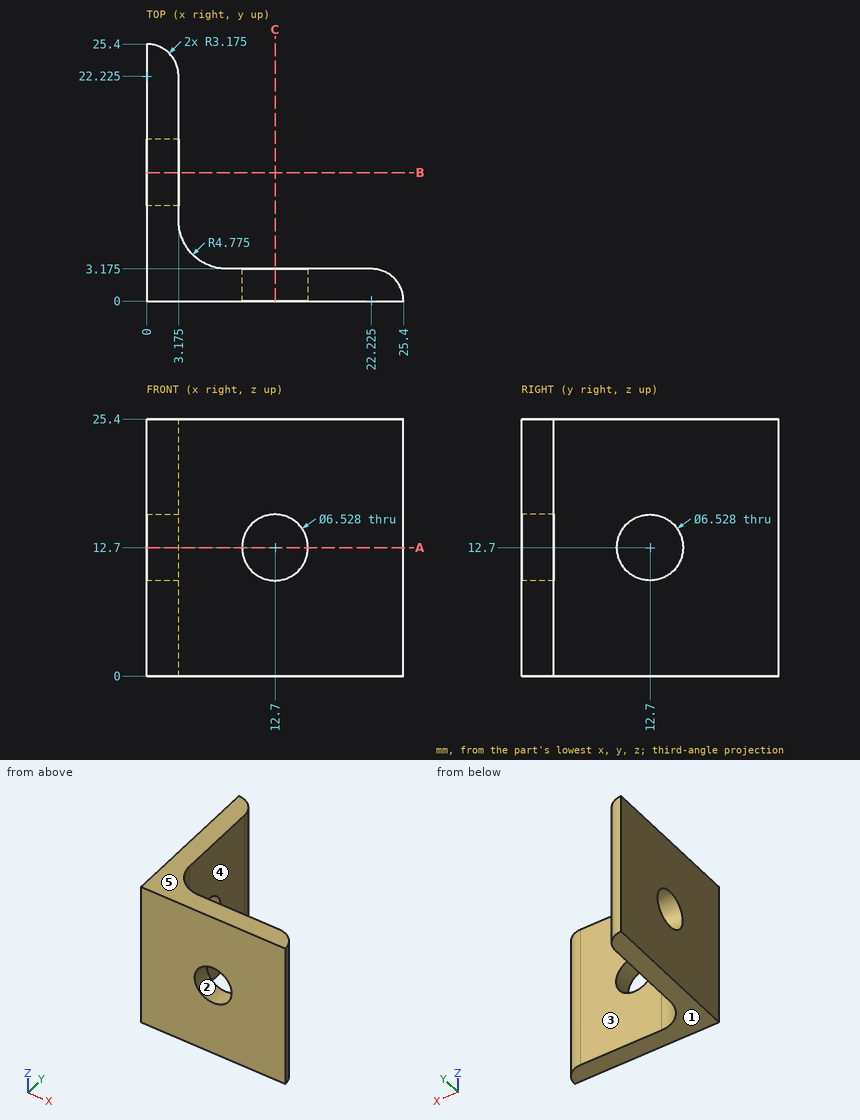
Could you check a few things on this drawing? It's one solid part, dimensions in mm from its lowest x, y, z. A direction names the side the tool comes from. Coordinates: 2 decimals unless noted, no trailing zeros. Loops run counter-clockwise (first coordinate to the right, second up) from the corner with the lowest first, then second, coordinate; pieces in that order, holes last.
1. For the marked faces 4 and 5, which set-ups out of +Z, -Z, +X, -X, +Y, -Y let a thin tool reach every point of the face, with its end or its side?
2. Imagine slicing it at B-B (y = 12.7). Please give me the cut outline in (x, z) (1 decimal).
3. I need wall thicknesses on L1, parallel to Z at x = 12.7, y = 2.15; L2, parallel to Y at x = 0.7, z = 12.7; L3, parallel to Y at x = 15.5, z = 18.5 (3 decimals). Which ranges of each line are inside material? Lowest first, please.
4. We'd pull the mould along Z, two halves only. Please class the marked faces 1, 2 and 3: released by +Z, released by -Z, zero draft, split by the parting line, or undercut.
5. For P1, Ø4.5, axis at x = 15.5, z = 17, coming from the +Y side (3 decimals); P2, Ø5, axis at y = 4.5, z = 9, coming from the +X side; P3, Ø8.5, axis at y = 12.7, z = 12.7, coming from the +X side (3 decimals), each with a flat end and sliding along its axis, tell me the tip position at first contact or that it passes through.
6. Imagine slicing it at A-A (z = 12.7). Give the number of separate pieces and of enclosed holes in the cut face, and give its area (3 significant figures).
Computed values:
1. face 4: +Z, -Z, +X, +Y
1. face 5: +Z, +X, -X, +Y, -Y
2. outline: (0, 0) - (3.2, 0) - (3.2, 9.4) - (0, 9.4) - close; (0, 16) - (3.2, 16) - (3.2, 25.4) - (0, 25.4) - close
3. L1: z = 0 to 9.44, 15.96 to 25.4
3. L2: y = 0 to 9.44, 15.96 to 25.32
3. L3: y = 0 to 3.175
4. face 1: released by -Z
4. face 2: undercut
4. face 3: zero draft
5. P1: stops at y = 3.175
5. P2: stops at x = 24.69
5. P3: stops at x = 3.175
6. separate pieces: 3
6. enclosed holes: 0
6. area: 110 mm2
